Model file for the job. Use its own axes, mm. Round coordinates to 2 decimals unless told otherwise and drop trailing zeros. Loops run counter-clockwise (first coordinate to the right, second up) from the corner with the lowest first, then second, coordinate; pieces in that order, holes last. Notation, with made-up numbers: M -8.75,76.25 L 27.25,76.25 A21 ccw 27.25,90.25 Z; hole C 75.5,11 d7. An arc over 180 degrees is marked long. Answer in a Markdown table with one row per item.
from build123d import *

# Parameters (mm, degrees)
SKETCH1_R                                            = 1.5
SKETCH1_W                                            = 100
SKETCH1_H                                            = 100
BOSS_EXTRUDE1_DEPTH                                  = 10
FILLET1_R                                            = 10
CSK_FOR_M4_HEX_SOCKET_COUNTERSUNK_CAP_SC_D           = 4.5
CSK_FOR_M4_HEX_SOCKET_COUNTERSUNK_CAP_SC_CSINK_D     = 8.96
CSK_FOR_M4_HEX_SOCKET_COUNTERSUNK_CAP_SC_CSINK_ANGLE = 90
SKETCH14_R                                           = 2.5
CUT_EXTRUDE1_DEPTH                                   = 8
FILLET2_R                                            = 45
M6_TAPPED_HOLE1_D                                    = 5
M3_TAPPED_HOLE2_D                                    = 2.5
M3_TAPPED_HOLE2_DEPTH                                = 21.5
M3_TAPPED_HOLE2_TIP                                  = 0.751075774
M3_TAPPED_HOLE1_D                                    = 2.5
M3_TAPPED_HOLE1_DEPTH                                = 21.5
M3_TAPPED_HOLE1_TIP                                  = 0.751075774
FILLET3_R                                            = 30


with BuildPart() as part:
    # Sketch1 → Boss-Extrude1 (new body)
    with BuildSketch(Plane(origin=(0, 0, 0), x_dir=(1, 0, 0), z_dir=(0, 1, 0))):
        Polygon((0, 0), (0, 160), (235, 160), (235, 95), (280, 95), (280, 65), (235, 65), (235, 0), align=None)
        with Locations(Location((50, 145, 0), (0, 0, 270))):
            Circle(SKETCH1_R, mode=Mode.SUBTRACT)
        with Locations(Location((50, 15, 0), (0, 0, 270))):
            Circle(SKETCH1_R, mode=Mode.SUBTRACT)
        with Locations(Location((250, 80, 0), (0, 0, 270))):
            Circle(SKETCH1_R, mode=Mode.SUBTRACT)
        with Locations((115, 80)):
            Rectangle(SKETCH1_W, SKETCH1_H, mode=Mode.SUBTRACT)
    extrude(amount=BOSS_EXTRUDE1_DEPTH)

    # Fillet1
    fillet1_edges = [part.edges().sort_by_distance(p)[0] for p in [
        (0, 5, 0),
        (0, 5, -160),
        (235, 5, -160),
        (235, 5, -95),
        (280, 5, -95),
        (280, 5, -65),
        (235, 5, -65),
        (235, 5, 0),
    ]]
    fillet(fillet1_edges, radius=FILLET1_R)

    # CSK for M4 Hex Socket Countersunk Cap Screw1 (through all)
    with Locations(Plane(origin=(0, 10, 0), x_dir=(1, 0, 0), z_dir=(0, 1, 0))):
        with Locations((170.65, 80), (180.65, 80), (195.65, 80), (210.65, 80), (170.65, 96), (170.65, 64)):
            CounterSinkHole(CSK_FOR_M4_HEX_SOCKET_COUNTERSUNK_CAP_SC_D / 2, CSK_FOR_M4_HEX_SOCKET_COUNTERSUNK_CAP_SC_CSINK_D / 2, counter_sink_angle=CSK_FOR_M4_HEX_SOCKET_COUNTERSUNK_CAP_SC_CSINK_ANGLE)

    # Sketch14 → Cut-Extrude1 (cut)
    with BuildSketch(Plane.XZ):
        with Locations(Location((270, -80, 0), (0, 0, 270))):
            Circle(SKETCH14_R)
        with Locations(Location((15, -15, 0), (0, 0, 270))):
            Circle(SKETCH14_R)
        with Locations(Location((15, -140, 0), (0, 0, 270))):
            Circle(SKETCH14_R)
    extrude(amount=-CUT_EXTRUDE1_DEPTH, mode=Mode.SUBTRACT)

    # Fillet2
    fillet2_edges = [part.edges().sort_by_distance(p)[0] for p in [
        (65, 5, -130),
        (65, 5, -30),
    ]]
    fillet(fillet2_edges, radius=FILLET2_R)

    # M6 Tapped Hole1 (through all)
    with Locations(Plane(origin=(0, 10, 0), x_dir=(1, 0, 0), z_dir=(0, 1, 0))):
        with Locations((50, 145), (250, 80), (50, 15)):
            Hole(M6_TAPPED_HOLE1_D / 2)

    # M3 Tapped Hole2
    with Locations(Plane(origin=(280, 5, -80), x_dir=(0, 0, 1), z_dir=(1, 0, 0))):
        with Locations((0, 0)):
            Hole(M3_TAPPED_HOLE2_D / 2, depth=M3_TAPPED_HOLE2_DEPTH)
            with Locations((0, 0, -(M3_TAPPED_HOLE2_DEPTH + M3_TAPPED_HOLE2_TIP / 2))):  # 118° drill point
                Cone(0, M3_TAPPED_HOLE2_D / 2, M3_TAPPED_HOLE2_TIP, mode=Mode.SUBTRACT)

    # M3 Tapped Hole1
    with Locations(Plane.ZY):
        with Locations((-140, 5), (-15, 5)):
            Hole(M3_TAPPED_HOLE1_D / 2, depth=M3_TAPPED_HOLE1_DEPTH)
            with Locations((0, 0, -(M3_TAPPED_HOLE1_DEPTH + M3_TAPPED_HOLE1_TIP / 2))):  # 118° drill point
                Cone(0, M3_TAPPED_HOLE1_D / 2, M3_TAPPED_HOLE1_TIP, mode=Mode.SUBTRACT)

    # Fillet3
    fillet3_edges = [part.edges().sort_by_distance(p)[0] for p in [
        (165, 5, -30),
        (165, 5, -130),
    ]]
    fillet(fillet3_edges, radius=FILLET3_R)


solid = part.part
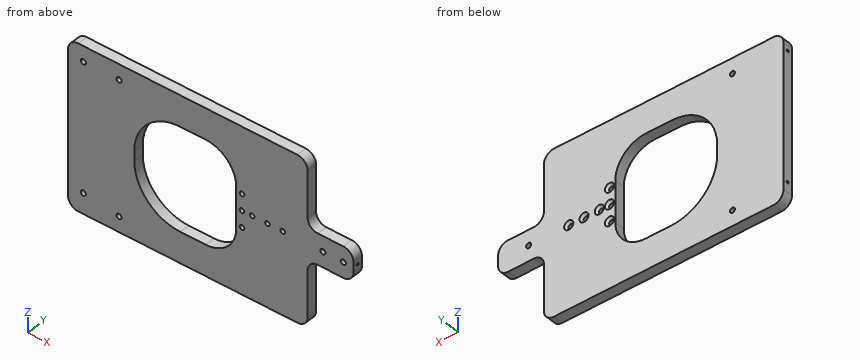
1. Saw through at A-A (z = -124.5). Write the cut outline in (x, y).
Verdict:
| item | result |
|---|---|
| outline | M 0,0 L 88.44,0 L 88.44,10 L 0,10 Z; M 152.31,0 L 235,0 L 235,10 L 152.31,10 Z |
2. Wall check: probe 1 along X at (y, z) = (0.75, -15); probe 2 along Z at (x, y) = (264.5, 5); probe 3 along Z at (x, y) = (108.5, 9.75) (3 decimals). Give the ranges that are in metal, low to high.
Verdict:
| item | result |
|---|---|
| probe 1 | x = 0 to 12.5, 17.5 to 47.5, 52.5 to 235 |
| probe 2 | z = -95 to -81.25, -78.75 to -65 |
| probe 3 | z = -160 to -129.975, -30.025 to 0 |
3. Pin check, flat tips, straight feed: pin 1 (1.5 mm diameter, centred on y = 5, z = -140, fed in from +X); pin 2 (5 mm diameter, centred on x = 238.5, y = 4, fed in from -Z); pin 3 (4 mm diameter, centred on x = 270, z = -80, fed in from -Y); pin 4 (3.5 mm diameter, centred on x = 180.65, z = -80, fed in from +Y). Stop position of each tip, or through.
Verdict:
| item | result |
|---|---|
| pin 1 | stops at x = 235 |
| pin 2 | stops at z = -100.64 |
| pin 3 | stops at y = 8 |
| pin 4 | passes through |
4. Saw through at B-B (y = 2). State how many separate pieces and enclosed holes the cut face has, and give its area (3 significant figures).
Verdict:
| item | result |
|---|---|
| separate pieces | 1 |
| enclosed holes | 13 |
| area | 29,900 mm² |
